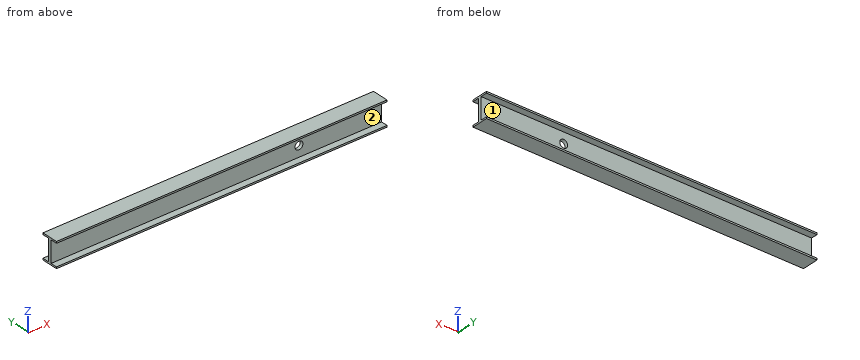
```python
from build123d import *

# Parameters (mm, degrees)
SKETCH1_W           = 200
SKETCH1_H           = 15
BOSS_EXTRUDE1_DEPTH = 10
CUT_EXTRUDE1_DEPTH  = 4
SKETCH4_W           = 200
SKETCH4_H           = 13
CUT_EXTRUDE2_DEPTH  = 4
SKETCH5_R           = 2.4
CUT_EXTRUDE3_DEPTH  = 10


with BuildPart() as part:
    # Sketch1 → Boss-Extrude1 (new body)
    with BuildSketch(Plane(origin=(0, 0, 0), x_dir=(1, 0, 0), z_dir=(0, 1, 0))):
        with Locations((22.463138005, -9.901926804)):
            Rectangle(SKETCH1_W, SKETCH1_H)
    extrude(amount=BOSS_EXTRUDE1_DEPTH)

    # Sketch3 → Cut-Extrude1 (cut)
    with BuildSketch(Plane(origin=(0, 10, 0), x_dir=(1, 0, 0), z_dir=(0, 1, 0))):
        Polygon((-77.536861995, -3.454668646), (-77.536861995, -16.401926804), (122.463138005, -16.401926804), (122.463138005, -3.541728885), (122.463138005, -3.401926804), (-77.536861995, -3.401926804), align=None)
    extrude(amount=-CUT_EXTRUDE1_DEPTH, mode=Mode.SUBTRACT)

    # Sketch4 → Cut-Extrude2 (cut)
    with BuildSketch(Plane.XZ):
        with Locations((22.463138005, 9.901926804)):
            Rectangle(SKETCH4_W, SKETCH4_H)
    extrude(amount=-CUT_EXTRUDE2_DEPTH, mode=Mode.SUBTRACT)

    # Sketch5 → Cut-Extrude3 (cut)
    with BuildSketch(Plane(origin=(0, 4, 0), x_dir=(-1, 0, 0), z_dir=(0, -1, 0))):
        with Locations((-72.463138005, -9.901926804)):
            Circle(SKETCH5_R)
    extrude(amount=-CUT_EXTRUDE3_DEPTH, mode=Mode.SUBTRACT)


solid = part.part
```
Here's how the part is built. I have some questions about the finished solid (model axes, mm). Face numbers are marked on the shaded views. A direction names the side the tool comes from. Coordinates: 2 decimals unless noted, no trailing zeros. Order: outer loops, then holes, each group sorted by start corner. A loop starts at its lowest first (then second) coordinate and runs counter-clockwise, first axis right, second up. Notation, with made-up numbers: (47, -34) - (65, -34) arc R6 ccw to (65, -26) - close; hole circle Ø11 at (89, -7). An arc over 180 degrees is marked (long way). One line per question, with ' | ' between items.
(1) Will these pins go through, and if not, where does the flat tip stop? pin 1 (4 mm diameter, centred on x = 47, z = 8.5, fed in from +Y); pin 2 (6 mm diameter, centred on y = 7.5, z = 5.5, fed in from -X); pin 3 (3 mm diameter, centred on x = 72.46, z = 9.9, fed in from +Y).
Report:
pin 1: stops at y = 6 | pin 2: stops at x = -77.54 | pin 3: passes through
(2) If I drill on L1, parallel to Z at x = 19.5, y = 1.5; L2, parallel to Y at x = -44.5, z = 7.75, over which ranges is the centre line in solid material (lowest first)?
Report:
L1: z = 2.4 to 3.4, 16.4 to 17.4 | L2: y = 4 to 6
(3) For the marked faces 1 and 2, which set-ups out of +Z, -Z, +X, -X, +Y, -Y let a thin tool reach every point of the face, with its end or its side?
Report:
face 1: +X, -X, +Y | face 2: +X, -X, -Y
(4) Suppose I cut it at A-A on y = 1.75. List the corners of the cut face in (x, z) for me.
Report:
outline: (-77.54, 2.4) - (122.46, 2.4) - (122.46, 3.4) - (-77.54, 3.4) - close; (-77.54, 16.4) - (122.46, 16.4) - (122.46, 17.4) - (-77.54, 17.4) - close
(5) Suppose I cut it at B-B on x = 94. List the corners of the cut face in (y, z) for me, and give its area (3 significant figures).
Report:
outline: (0, 2.4) - (10, 2.4) - (10, 3.4) - (6, 3.4) - (6, 16.4) - (10, 16.4) - (10, 17.4) - (0, 17.4) - (0, 16.4) - (4, 16.4) - (4, 3.4) - (0, 3.4) - close | area: 46.0 mm2
